Input: part model. Units: mm. Frame: model coordinates. A direction names the side the tool comes from. Give positions to 0.01 mm unless a question says otherwise; leave off trailing zeros. Order: outer loops, then holes, each group sorted by start corner. A loop starts at its lowest first (then second) coordinate and runs counter-clockwise, first axis right, second up. Notation, with made-up numbers: (12.25, 75) - (48.25, 75) arc R31 cw to (48.25, 103) - close; hole circle Ø4 at (34.25, 7.5). An arc over 180 degrees is marked (long way). Answer in a Markdown table with one row per item. Add a question column.
from build123d import *

# Parameters (mm, degrees)
SALIENTE_EXTRUIR1_DEPTH = 2.125
CROQUIS2_R              = 5
SALIENTE_EXTRUIR2_DEPTH = 2.5
REDONDEO1_R             = 1.625
SKETCH1_R               = 2.45
CUT_EXTRUDE1_DEPTH      = 3.1
CHAMFER1_SIZE           = 2.125
CUT_EXTRUDE2_DEPTH      = 68.459362768
CUT_EXTRUDE2_DEPTH_BACK = 68.459362768
SKETCH2_W               = 5
SKETCH2_H               = 28.351341624
CUT_EXTRUDE3_DEPTH      = 68.002686513
CUT_EXTRUDE3_DEPTH_BACK = 68.002686513
SKETCH3_R               = 1.05
CUT_EXTRUDE4_DEPTH      = 68.459362768
CUT_EXTRUDE4_DEPTH_BACK = 2.125


# Some blends are built 0.0001 mm under size
with BuildPart() as part:
    # Croquis1 → Saliente-Extruir1 (new, symmetric)
    with BuildSketch(Plane.XY):
        Polygon((60, 0), (-60, 0), (-40, 30), (40, 30), align=None)
    extrude(amount=SALIENTE_EXTRUIR1_DEPTH, both=True)

    # Croquis2 → Saliente-Extruir2 (add)
    with BuildSketch(Plane.XZ):
        with Locations(Location((0, 0, 0), (0, 0, 25.150663413))):
            Circle(CROQUIS2_R)
    extrude(amount=SALIENTE_EXTRUIR2_DEPTH)

    # Redondeo1
    # the kernel refuses this fillet: 1.625 mm, written as the material it adds along each edge
    with BuildSketch(Plane(origin=(8.588466748, 0, -2.125), x_dir=(0, 1, 0), z_dir=(-1, 0, 0))) as redondeo1_piece_1_section:
        with BuildLine():
            CenterArc((REDONDEO1_R, REDONDEO1_R), REDONDEO1_R, 180, 90)
            Line((0, REDONDEO1_R), (0, 0))
            Line((0, 0), (REDONDEO1_R, 0))
        make_face()
    redondeo1_piece_1 = extrude(amount=17.176933495, mode=Mode.PRIVATE)
    redondeo1_piece_1 = redondeo1_piece_1 & Plane(origin=(0, 0.370660795, 0), x_dir=(0.9051933495081991, 0, 0.4250000000072087), z_dir=(0, 1, 0)) * Cylinder(5, 41, mode=Mode.PRIVATE)
    add(redondeo1_piece_1)
    with BuildSketch(Plane(origin=(8.588466748, 0, 2.125), x_dir=(0, 1, 0), z_dir=(-1, 0, 0))) as redondeo1_piece_2_section:
        with BuildLine():
            CenterArc((REDONDEO1_R, -REDONDEO1_R), REDONDEO1_R, 90, 90)
            Line((0, -REDONDEO1_R), (0, 0))
            Line((0, 0), (REDONDEO1_R, 0))
        make_face()
    redondeo1_piece_2 = extrude(amount=17.176933495, mode=Mode.PRIVATE)
    redondeo1_piece_2 = redondeo1_piece_2 & Plane(origin=(0, 0.370660827, 0), x_dir=(0.9051933495081991, 0, 0.4250000000072087), z_dir=(0, 1, 0)) * Cylinder(5, 41, mode=Mode.PRIVATE)
    add(redondeo1_piece_2)

    # Sketch1 → Cut-Extrude1 (cut)
    with BuildSketch(Plane.XZ.offset(2.5)):
        with Locations(Location((0, 0, 0), (0, 0, 270))):
            Circle(SKETCH1_R)
    extrude(amount=-CUT_EXTRUDE1_DEPTH, mode=Mode.SUBTRACT)

    # Chamfer1
    chamfer1_edges = [part.edges().sort_by_distance(p)[0] for p in [
        (50, 15, -2.125),
        (0, 30, -2.125),
        (-50, 15, -2.125),
        (50, 15, 2.125),
        (0, 30, 2.125),
        (-50, 15, 2.125),
    ]]
    chamfer(chamfer1_edges, length=CHAMFER1_SIZE - 0.0001)  # a hair under: the kernel refuses the full size

    # Sketch2 → Cut-Extrude2 (cut, two sides: drawn at the far end of the back side and taken through both)
    with BuildSketch(Plane.XY.offset(2.125).offset(-CUT_EXTRUDE2_DEPTH_BACK)):
        with Locations((0, 15.85)):
            Rectangle(SKETCH2_W, SKETCH2_H)
    extrude(amount=CUT_EXTRUDE2_DEPTH + CUT_EXTRUDE2_DEPTH_BACK, mode=Mode.SUBTRACT)

    # Sketch3 → Cut-Extrude3 (cut, two sides: drawn at the far end of the back side and taken through both)
    with BuildSketch(Plane.XZ.offset(-0.6).offset(-CUT_EXTRUDE3_DEPTH_BACK)):
        with Locations(Location((0, 0, 0), (0, 0, 270))):
            Circle(SKETCH3_R)
    extrude(amount=CUT_EXTRUDE3_DEPTH + CUT_EXTRUDE3_DEPTH_BACK, mode=Mode.SUBTRACT)

    # Sketch4 → Cut-Extrude4 (cut, two sides: drawn at the far end of the back side and taken through both)
    with BuildSketch(Plane.XY.offset(2.125).offset(-CUT_EXTRUDE4_DEPTH_BACK)):
        with BuildLine():
            Line((2.5, 25.918582297), (2.5, 19.918582297))
            Line((2.5, 19.918582297), (6.5, 19.918582297))
            ThreePointArc((6.5, 19.918582297), (9.5, 22.918582297), (6.5, 25.918582297))
            Line((6.5, 25.918582297), (2.5, 25.918582297))
        make_face()
        with BuildLine():
            Line((6.5, 11.755746891), (2.5, 11.755746891))
            Line((2.5, 11.755746891), (2.5, 5.755746891))
            Line((2.5, 5.755746891), (6.5, 5.755746891))
            ThreePointArc((6.5, 5.755746891), (9.5, 8.755746891), (6.5, 11.755746891))
        make_face()
        with BuildLine():
            Line((-6.5, 19.918582297), (-2.5, 19.918582297))
            Line((-2.5, 19.918582297), (-2.5, 25.918582297))
            Line((-2.5, 25.918582297), (-6.5, 25.918582297))
            ThreePointArc((-6.5, 25.918582297), (-9.5, 22.918582297), (-6.5, 19.918582297))
        make_face()
        with BuildLine():
            Line((-2.5, 5.755746891), (-2.5, 11.755746891))
            Line((-2.5, 11.755746891), (-6.5, 11.755746891))
            ThreePointArc((-6.5, 11.755746891), (-9.5, 8.755746891), (-6.5, 5.755746891))
            Line((-6.5, 5.755746891), (-2.5, 5.755746891))
        make_face()
    extrude(amount=CUT_EXTRUDE4_DEPTH + CUT_EXTRUDE4_DEPTH_BACK, mode=Mode.SUBTRACT)


solid = part.part
Q1. Section A-A, the plane x = 0. Return loops of the section in (y, z) (3 decimals), then the cut area to 3 significant figures.
Q2. Access query for faces 1 (the flat face through (2.5, 16, -1)), 2 (the cylindrical face through (0.736, -0.972, -2.337)), 3 (the flat face through (5, 11.756, 1)), 4 (the flat face through (48.988, 14.629, 1.048)). Directions: +Z, -Z, +X, -X, +Y, -Y. A direction counts if a zero-diameter tool reaches every point of the face in a straight line with its end or side. Return the directions, or none.
Q3. Contact query for flat-ended pins moving along their axis: P1, Ø1.8, axis at x = 4.5, y = 22, coming from the +Z side; P2, Ø1.3, axis at y = 11.5, z = 0, coming from the -X side; P3, Ø5, axis at x = 32.5, z = -1, coming from the -Y side; P4, Ø4, axis at x = 5, z = -1.5, coming from the -Y side. Output: stop coordinate, or through.
Q4. Pull-direction query (Z, two-part tool) for faces 5 (the flat face through (-4, 25.919, 1)), 6 (the flat face through (21, 29, 1)), 7 (the flat face through (-1, 0.6, -1)); classes: +Z half, -Z half, draft (parallel to the pull), parting line (faces both ways), or undercut.
Q5. Line query: probe 1 along X at (y, z) = (-0.7, 0); probe 2 along Z at (x, y) = (-44, 15.5) (3 decimals); probe 3 along Y at (x, z) = (-2, 1.5). Output: solid intervals per line, ascending.
Computed:
| question | item | result |
|---|---|---|
| 1 | outline | (-2.5, -5) - (0, -5) - (0, -3.75) arc R1.625 cw to (1.625, -2.125) - (1.674, -2.125) - (1.674, -1.05) - (0.6, -1.05) - (0.6, -2.45) - (-2.5, -2.45) - close; (-2.5, 2.45) - (0.6, 2.45) - (0.6, 1.05) - (1.674, 1.05) - (1.674, 2.125) - (1.625, 2.125) arc R1.625 cw to (0, 3.75) - (0, 5) - (-2.5, 5) - close |
| 1 | area | 15.8 mm^2 |
| 2 | face 1 | +Z, -Z, +Y |
| 2 | face 2 | -Y |
| 2 | face 3 | +Z |
| 2 | face 4 | +Z, +X, +Y |
| 3 | P1 | stops at z = 0 |
| 3 | P2 | stops at x = -52.77 |
| 3 | P3 | stops at y = 0 |
| 3 | P4 | stops at y = -2.5 |
| 4 | face 5 | draft |
| 4 | face 6 | +Z half |
| 4 | face 7 | undercut |
| 5 | probe 1 | x = -5 to -2.45, 2.45 to 5 |
| 5 | probe 2 | z = -2.125 to 2.125 |
| 5 | probe 3 | y = -2.5 to 1.67 |
